Input: part model. Units: mm. Frame: model coordinates. Face numbers are marked on the shaded views. Coordinates: 2 decimals unless noted, no trailing zeros. Loops run counter-clockwise (first coordinate to the right, second up) from the corner with the lowest first, then second, coordinate; pieces in that order, holes last. Notation, with made-up numbers: (79.5, -16.5) -> (92.5, -16.5) arc R36 ccw to (92.5, 19.5) -> close; hole circle Ø1 at (37.25, 78.5). An arc over 180 degrees is marked (long way). Put each result on its own line as item: value. Start each with the question number.
1) Material intervals for L1, parallel to X at y = 8, z = 0; L2, parallel to Z at x = -4, y = 2; L3, parallel to Z at x = -6.5, y = 16.25, sorted ascending.
2) Cut plane D-D (y = 17.5). Return the cut outline in (x, z), plus the area to 3 significant figures.
3) Pull-direction query (X, two-part tool) for the marked faces 1, 2 and 3; classes: pulls with the +X half, pulls with the -X half, needs draft (parallel to the pull), parting line crosses it, or undercut.
4) Cut plane A-A (x = 0). Return the cut outline in (y, z).
5) Cut plane C-C (y = 13.75). Return the cut outline in (x, z), plus the area to 3 significant figures.
6) Cut plane B-B (z = 0). Return the cut outline in (x, y).
7) Contact query for flat-ended pins moving along their axis: P1, Ø2, axis at y = 14, z = -1.5, coming from the -X side; P2, Ø4, axis at y = 16.5, z = -6, coming from the +X side; P3, Ø1.5, axis at x = -5.5, y = 16.5, coming from the -Z side. Output: stop coordinate, or through.
from build123d import *

# Parameters (mm, degrees)
SKETCH1_R           = 10
BOSS_EXTRUDE1_DEPTH = 20
CUT_EXTRUDE1_REACH  = 26.495
SKETCH2_R           = 7.5
FILLET1_R           = 3


with BuildPart() as part:
    # Sketch1 → Boss-Extrude1 (new body)
    with BuildSketch(Plane(origin=(0, 0, 0), x_dir=(1, 0, 0), z_dir=(0, 1, 0))):
        with Locations(Location((0, 0, 0), (0, 0, 270))):
            Circle(SKETCH1_R)
    extrude(amount=BOSS_EXTRUDE1_DEPTH)

    # Sketch2 → Cut-Extrude1 (cut, up to next)
    with BuildSketch(Plane(origin=(0, 20, 0), x_dir=(1, 0, 0), z_dir=(0, 1, 0)), mode=Mode.PRIVATE) as cut_extrude1_sk1:
        with Locations(Location((0, 0, 0), (0, 0, 270))):
            Circle(SKETCH2_R)
    cut_extrude1_tool1 = extrude(cut_extrude1_sk1.sketch, amount=-CUT_EXTRUDE1_REACH, mode=Mode.PRIVATE) & part.part
    add(cut_extrude1_tool1.solids().sort_by_distance((0, 20, 0))[0], mode=Mode.SUBTRACT)

    # Fillet1
    # the kernel refuses this fillet: 3 mm, written as the material it takes off along each edge
    with BuildSketch(Plane(origin=(0, 20, 0), x_dir=(-1.8e-16, 0, 1), z_dir=(-1, 0, -1.8e-16))) as fillet1_piece_1:
        with BuildLine():
            CenterArc((10.5, -2.958039891550115), FILLET1_R, 99.5940682268595, 80.4059317731405)
            Line((7.5, -2.958039891550115), (7.44, -2.958039891550115))
            Line((7.44, -2.958039891550115), (7.44, 0))
            Line((7.44, 0), (7.5, 0.05999999999999872))
            ThreePointArc((7.5, 0.05999999999999872), (8.750000000000025, 0.05999999999999872), (9.99000000000005, 0.05916079783069961))
            Line((9.99000000000005, 0.05916079783069961), (10.00000000000005, -2.9843e-13))
        make_face()
    revolve(axis=Axis((0, 20, 0), (0, 1, 0)), mode=Mode.SUBTRACT)


solid = part.part
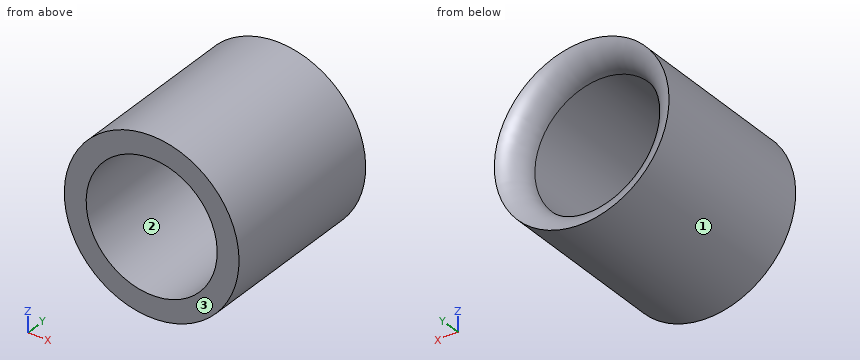
Results found:
1. L1: x = -10 to -7.5, 7.5 to 10
1. L2: z = -9.17 to -6.34, 6.34 to 9.17
1. L3: z = -7.6 to -3.74, 3.74 to 7.6
2. outline: circle Ø20 at (0, 0); hole circle Ø15.07 at (0, 0)
2. area: 136 mm2
3. face 1: parting line crosses it
3. face 2: undercut
3. face 3: needs draft
4. outline: (0, -10) -> (20, -10) arc R3 ccw to (17.04, -7.5) -> (0, -7.5) -> close; (0, 7.5) -> (17.04, 7.5) arc R3 ccw to (20, 10) -> (0, 10) -> close
5. outline: circle Ø20 at (0, 0); hole circle Ø15 at (0, 0)
5. area: 137 mm2
6. outline: (-10, 0) -> (-7.5, 0) -> (-7.5, 17.04) arc R3 ccw to (-10, 20) -> close; (7.5, 0) -> (10, 0) -> (10, 20) arc R3 ccw to (7.5, 17.04) -> close
7. P1: stops at x = -9.99
7. P2: stops at x = 9.17
7. P3: stops at z = -8.8
